For this review, take the finished solid that the model builds, in its own axes (mm). A direction names the side the tool comes from. Give positions to 0.01 mm unless a question says otherwise; leave off trailing zeros. Write each loop counter-clockwise with the first axis right and the second up, starting at its lowest first coordinate (ties: lowest second). Pieces come first, ordered by that corner, then holes. Notation, with made-up numbers: (59, -27.75) -> (102, -27.75) arc R23 ccw to (102, 11.25) -> close; hole circle Ø1 at (23.5, 35.5). An arc over 180 degrees is marked (long way). Return JSON: item names as keys, results as strings.
from build123d import *

# Parameters (mm, degrees)
BASE_FLANGE1_DEPTH        = 101.6
CHAMFER1_SIZE             = 25.4
FILLET1_R                 = 9.525
M10_CLEARANCE_HOLE1_D     = 11
M10_CLEARANCE_HOLE1_DEPTH = 57.658
M10_CLEARANCE_HOLE1_TIP   = 3.304733405
CHAMFER2_SIZE             = 1.27


# Sheet-metal steps are written as plain solids
with BuildPart() as part:
    # Sketch1 → Base-Flange1 (new body)
    with BuildSketch(Plane.XY):
        with BuildLine():
            Line((0, 39.116), (0, 0.7366))
            ThreePointArc((0, 0.7366), (0.215745145, 0.215745145), (0.7366, 0))
            Line((0.7366, 0), (50.0634, 0))
            ThreePointArc((50.0634, 0), (50.584254855, 0.215745145), (50.8, 0.7366))
            Line((50.8, 0.7366), (50.8, 39.116))
            Line((50.8, 39.116), (54.2163, 39.116))
            Line((54.2163, 39.116), (54.2163, 0.7366))
            ThreePointArc((54.2163, 0.7366), (52.999943752, -2.199943752), (50.0634, -3.4163))
            Line((50.0634, -3.4163), (0.7366, -3.4163))
            ThreePointArc((0.7366, -3.4163), (-2.199943752, -2.199943752), (-3.4163, 0.7366))
            Line((-3.4163, 0.7366), (-3.4163, 39.116))
            Line((-3.4163, 39.116), (0, 39.116))
        make_face()
    extrude(amount=BASE_FLANGE1_DEPTH)

    # Chamfer1
    chamfer1_edges = [part.edges().sort_by_distance(p)[0] for p in [
        (-1.70815, 39.116, 0),
        (52.50815, 39.116, 0),
        (-1.70815, 39.116, 101.6),
        (52.50815, 39.116, 101.6),
    ]]
    chamfer(chamfer1_edges, length=CHAMFER1_SIZE)

    # Fillet1
    fillet1_edges = [part.edges().sort_by_distance(p)[0] for p in [
        (52.50815, 13.716, 0),
        (52.50815, 39.116, 76.2),
        (52.50815, 39.116, 25.4),
        (52.50815, 13.716, 101.6),
        (-1.70815, 13.716, 0),
        (-1.70815, 39.116, 76.2),
        (-1.70815, 39.116, 25.4),
        (-1.70815, 13.716, 101.6),
    ]]
    fillet(fillet1_edges, radius=FILLET1_R)

    # M10 Clearance Hole1
    with Locations(Plane(origin=(54.2163, 0, 0), x_dir=(0, 0, -1), z_dir=(1, 0, 0))):
        with Locations((-50.8, 20.066)):
            Hole(M10_CLEARANCE_HOLE1_D / 2, depth=M10_CLEARANCE_HOLE1_DEPTH)
            with Locations((0, 0, -(M10_CLEARANCE_HOLE1_DEPTH + M10_CLEARANCE_HOLE1_TIP / 2))):  # 118° drill point
                Cone(0, M10_CLEARANCE_HOLE1_D / 2, M10_CLEARANCE_HOLE1_TIP, mode=Mode.SUBTRACT)

    # Chamfer2
    chamfer2_edges = [part.edges().sort_by_distance(p)[0] for p in [
        (-3.4163, 20.066, 45.3),
        (54.2163, 20.066, 45.3),
    ]]
    chamfer(chamfer2_edges, length=CHAMFER2_SIZE)


solid = part.part
1. Add section B-B, the plane z = 50.8. State the section outline as (x, y) points, plus the area to 3 significant figures.
Results found:
{"outline": "(-3.42, 0.74) arc R4.15 ccw to (0.74, -3.42) -> (50.06, -3.42) arc R4.15 ccw to (54.22, 0.74) -> (54.22, 13.3) -> (52.95, 14.57) -> (50.8, 14.57) -> (50.8, 0.74) arc R0.74 cw to (50.06, 0) -> (0.74, 0) arc R0.74 cw to (0, 0.74) -> (0, 14.57) -> (-2.15, 14.57) -> (-3.42, 13.3) -> close; (-3.42, 26.84) -> (-2.15, 25.57) -> (0, 25.57) -> (0, 39.12) -> (-3.42, 39.12) -> close; (50.8, 25.57) -> (52.95, 25.57) -> (54.22, 26.84) -> (54.22, 39.12) -> (50.8, 39.12) -> close", "area": "379 mm²"}
2. To check wall thickness, follow probe 1 along X at (y, z) = (32, 56); probe 2 along Y at (x, z) = (13.5, 63.5); probe 3 along Y at (x, z) = (52.5, 50.8). State the ranges of each line that lie inside material, in increasing order.
Results found:
{"probe 1": "x = -3.42 to 0, 50.8 to 54.22", "probe 2": "y = -3.42 to 0", "probe 3": "y = -2.63 to 14.57, 25.57 to 39.12"}
3. Add section C-C, the plane x = 20. State the section outline as (y, z) points.
Results found:
{"outline": "(-3.42, 0) -> (0, 0) -> (0, 101.6) -> (-3.42, 101.6) -> close"}
4. For pin 1 (8 mm diameter, centred on x = 22, z = 29, fed in from +Y); pin 2 (14.5 mm diameter, centred on y = 20.066, z = 50.8, fed in from -X), all flat-tipped, find the tip position at first contact; note any pin that passes through.
Results found:
{"pin 1": "stops at y = 0", "pin 2": "stops at x = -3.42"}
5. For faces 1 (the flat face through (0, 12, 50)), 2 (the flat face through (26, -1, 101.6)), list the 3-axis set-ups (+Z, -Z, +X, -X, +Y, -Y) from which the entire face can be reached by the end or side of a thin tool; tool diameter is ignored.
Results found:
{"face 1": "+Z, -Z, +Y", "face 2": "+Z, +X, -X, +Y, -Y"}
6. Add section A-A, the plane y = 3. State the section outline as (x, z) points, plus the area to 3 significant figures.
Results found:
{"outline": "(-3.42, 0) -> (0, 0) -> (0, 101.6) -> (-3.42, 101.6) -> close; (50.8, 0) -> (54.22, 0) -> (54.22, 101.6) -> (50.8, 101.6) -> close", "area": "694 mm²"}
7. Add section D-D, the plane y = 11.5. State the section outline as (x, z) points, plus the area to 3 significant figures.
Results found:
{"outline": "(-3.42, 0.16) -> (0, 0.16) -> (0, 101.44) -> (-3.42, 101.44) -> close; (50.8, 0.16) -> (54.22, 0.16) -> (54.22, 101.44) -> (50.8, 101.44) -> close", "area": "692 mm²"}
8. The part is to be moulded in two halves that separate along X. For faces 3 (the flat face through (25, 0, 50)), 4 (the cylindrical face through (-1.68, 38.41, 25.75)), 5 (the flat face through (54.216, 12, 50)), say which applies: +X half, -X half, draft (parallel to the pull), parting line (faces both ways), or undercut.
Results found:
{"face 3": "undercut", "face 4": "draft", "face 5": "+X half"}
